Build history of the part. All positions in model axes, mm. A direction names the side the tool comes from. Round coordinates to 2 decimals unless told otherwise and drop trailing zeros. Write each loop counter-clockwise with the first axis right and the second up, starting at its lowest first coordinate (ties: lowest second). Pieces come first, ordered by that corner, then holes. Notation, with made-up numbers: (80, 14.25) - (98, 14.25) arc R7 ccw to (98, 19.25) - close; hole circle Ø4 at (-33.5, 2). An arc over 180 degrees is marked (long way). Answer as a JSON object with one key per item and string values. Group by question number.
Item 1: Slice it at A-A, the plane y = 0. List the corners of the cut face in (x, z), then the cut area to 3 significant figures.
Item 2: Slice it at B-B, the plane z = -2.5. List the corners of the cut face in (x, y), then the cut area to 3 significant figures.
Item 3: Which spindle directions (+Z, -Z, +X, -X, +Y, -Y) get a long thin tool onto all of the face, cutting with end or side? Do faces 1 (the flat face through (0.489, -0.863, -0.64)), 2 (the flat face through (0, 0, -11.379)). Say none if no direction does.
Item 4: Flat gauge pins, fed straight in: pin 1 (1.5 mm diameter, centred on x = 0.5, z = -5.5, fed in from +Y); pin 2 (1.5 mm diameter, centred on x = -0.5, y = 1, fed in from +Z); pin 3 (2 mm diameter, centred on x = 2.5, y = 2.5, fed in from +Z); pin 4 (2 mm diameter, centred on x = -1.5, z = -7.5, fed in from +Y). Where does each tip first touch, or does it go through?
Item 5: Slice it at C-C, the plane x = -2.5. List the corners of the cut face in (y, z).
Item 6: Two-plate mould, pull along X, no slides. Class faces 3 (the flat face through (1.4, -1.4, -1.854)), 4 (the cylindrical face through (-0.53, 1.67, -6.38)), 5 (the flat face through (0.503, 0.855, -0.64)): +X half, -X half, draft (parallel to the pull), parting line (faces both ways), or undercut.
Item 7: Probe line 1 (X direction, y = 0, z = -5); line 2 (Z direction, x = 0.75, y = 0.5); line 3 (X direction, y = -1.5, z = -6.5). List the from-to ranges inside material, lowest first. Write a range as from..to.
from build123d import *

# Parameters (mm, degrees)
SKETCH1_W          = 9.525
SKETCH1_H          = 1.7526
CHAMFER1_SIZE      = 0.5953125
CUT_EXTRUDE2_DEPTH = 1.29794


with BuildPart() as part:
    # Sketch1 → Revolve1 (revolve)
    with BuildSketch(Plane(origin=(0, 0, 0), x_dir=(0, 0, -1), z_dir=(1, 0, 0))):
        with Locations((6.6167, 0.8763)):
            Rectangle(SKETCH1_W, SKETCH1_H)
    revolve(axis=Axis((0, 0, -11.3792), (0, 0, 1)))

    # Chamfer1
    chamfer1_edges = [part.edges().sort_by_distance(p)[0] for p in [
        (0, -1.7526, -11.3792),
    ]]
    chamfer(chamfer1_edges, length=CHAMFER1_SIZE)

    # Sketch7 → Revolve2 (revolve)
    with BuildSketch(Plane(origin=(0, 0, 0), x_dir=(0, 0, -1), z_dir=(1, 0, 0)), mode=Mode.PRIVATE) as revolve2_sk:
        with BuildLine():
            Line((1.57607, 3.3274), (1.8542, 3.3274))
            Line((1.8542, 3.3274), (1.8542, 0))
            Line((1.8542, 0), (0, 0))
            Line((0, 0), (0, 1.7526))
            ThreePointArc((0, 1.7526), (0.668695369, 2.659435873), (1.57607, 3.3274))
        make_face()
    revolve(revolve2_sk.sketch.rotate(Axis((0, 0, 0), (0, 0, -1)), 180), axis=Axis((0, 0, 0), (0, 0, -1)))

    # Sketch5 → Cut-Extrude2 (cut)
    with BuildSketch(Plane.XY):
        Polygon((0.9921875, -0.57283972), (0.9921875, 0.57283972), (0, 1.14567944), (-0.9921875, 0.57283972), (-0.9921875, -0.57283972), (0, -1.14567944), align=None)
    extrude(amount=-CUT_EXTRUDE2_DEPTH, mode=Mode.SUBTRACT)

    # Cut-Extrude3 cone 1 section (on through the dimple's axis) → Cut-Extrude3 (revolve, cut)
    with BuildSketch(Plane(origin=(0, 0, 0), x_dir=(0, -1, 0), z_dir=(1, 0, 0))):
        Polygon((0, 0), (1.14567944, 0), (0, 1.14567944), align=None)
    revolve(axis=Axis((0, 0, 0), (0, 0, -1)), mode=Mode.SUBTRACT)


solid = part.part
Geometry says:
{
 "1": {"outline": "(-3.33, -1.85) - (-1.75, -1.85) - (-1.75, -10.78) - (-1.16, -11.38) - (1.16, -11.38) - (1.75, -10.78) - (1.75, -1.85) - (3.33, -1.85) - (3.33, -1.58) arc R3.76 ccw to (1.75, 0) - (1.15, 0) - (0.99, -0.15) - (0.99, -1.3) - (-0.99, -1.3) - (-0.99, -0.15) - (-1.15, 0) - (-1.75, 0) arc R3.76 ccw to (-3.33, -1.58) - close", "area": "40.8 mm^2"},
 "2": {"outline": "circle Ø3.51 at (0, 0)", "area": "9.65 mm^2"},
 "3": {"face 1": "+Z", "face 2": "-Z, +X, -X, +Y, -Y"},
 "4": {"pin 1": "stops at y = 1.75", "pin 2": "stops at z = 0", "pin 3": "stops at z = -0.55", "pin 4": "stops at y = 1.68"},
 "5": {"outline": "(-2.2, -1.85) - (2.2, -1.85) - (2.2, -1.58) arc R2.81 ccw to (-2.2, -1.58) - close"},
 "6": {"face 3": "draft", "face 4": "parting line", "face 5": "undercut"},
 "7": {"line 1": "x = -1.75..1.75", "line 2": "z = -11.38..-1.3", "line 3": "x = -0.91..0.91"}
}
